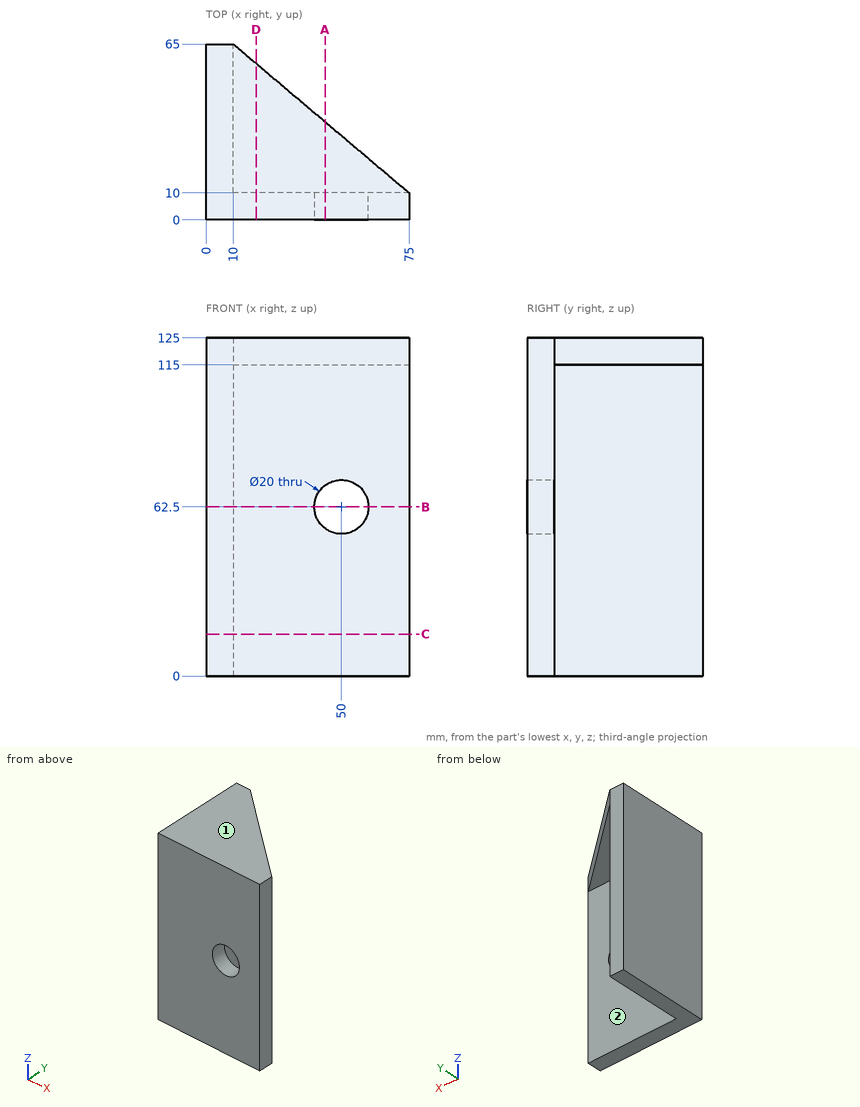
Here's the drawing with two shaded views (mm, measured from the low corner). I have some questions. A direction names the side the tool comes from. Coordinates: 2 decimals unless noted, no trailing zeros. Write each loop counter-clockwise with the first axis right and the second up, starting at its lowest first coordinate (ties: lowest second). Pieces come first, ordered by that corner, then holes. Notation, with made-up numbers: (75, -37) -> (125, -37) arc R7 cw to (125, -28) -> close; hole circle Ø4 at (36.25, -24.75). An arc over 180 degrees is marked (long way). Write item = value, one per line. Start each with the question number.
(1) Which directions (+Z, -Z, +X, -X, +Y, -Y) give clear straight access to the entire face, cutting with the end or side of a thin tool? Please do the marked faces 1 and 2.
(2) I want a section at B-B (z = 62.5). Please give me the cut outline in (x, y), plus the area to 3 significant figures.
(3) I want a section at C-C (z = 15.5). Please give me the cut outline in (x, y), plus the area to 3 significant figures.
(4) Will these pins go through, and if not, where does the flat tip stop? pin 1 (1 mm diameter, centred on x = 54.5, z = 26, fed in from +Y); pin 2 (10 mm diameter, centred on x = 34.5, y = 38, fed in from -Z).
(5) I want a section at A-A (x = 44). Please give me the cut outline in (y, z), plus the area to 3 significant figures.
(6) I want a section at D-D (x = 18.5). Please give me the cut outline in (y, z).
(7) I need wall thicknesses on line 1 (X direction, y = 5, z = 62); line 2 (Z direction, x = 50, y = 7.25); line 3 (X direction, y = 46, z = 54). Which ranges of each line are inside material? Lowest first, please. Write a range as [from, to].
Result set:
q1.face_1 = +Z, +X, -X, +Y, -Y
q1.face_2 = -Z, +X, +Y
q2.outline = (0, 0) -> (40, 0) -> (40, 10) -> (10, 10) -> (10, 65) -> (0, 65) -> close; (60, 0) -> (75, 0) -> (75, 10) -> (60, 10) -> close
q2.area = 1,100 mm2
q3.outline = (0, 0) -> (75, 0) -> (75, 10) -> (10, 10) -> (10, 65) -> (0, 65) -> close
q3.area = 1,300 mm2
q4.pin_1 = 10
q4.pin_2 = 115
q5.outline = (0, 0) -> (10, 0) -> (10, 54.5) -> (0, 54.5) -> close; (0, 70.5) -> (10, 70.5) -> (10, 115) -> (36.23, 115) -> (36.23, 125) -> (0, 125) -> close
q5.area = 1,350 mm2
q6.outline = (0, 0) -> (10, 0) -> (10, 115) -> (57.81, 115) -> (57.81, 125) -> (0, 125) -> close
q7.line_1 = [0, 40.01], [59.99, 75]
q7.line_2 = [0, 52.5], [72.5, 125]
q7.line_3 = [0, 10]
